Input: dimensioned drawing with shaded views. Units: mm. Origin: part minimum x, y, z. A direction names the side the tool comes from. Give positions to 0.01 mm unless a question says otherwise; leave off trailing zeros. Order: outer loops, then holes, each group sorted by start corner. A loop starts at its lowest first (then second) coordinate and runs counter-clockwise, first axis right, second up. Notation, with made-up numbers: (73, 58.5) - (117, 58.5) arc R25 cw to (117, 97.5) - close; hole circle Ø4 at (-14, 19.5). An arc over 180 degrees is marked (long way). Use a Markdown table: item, result.
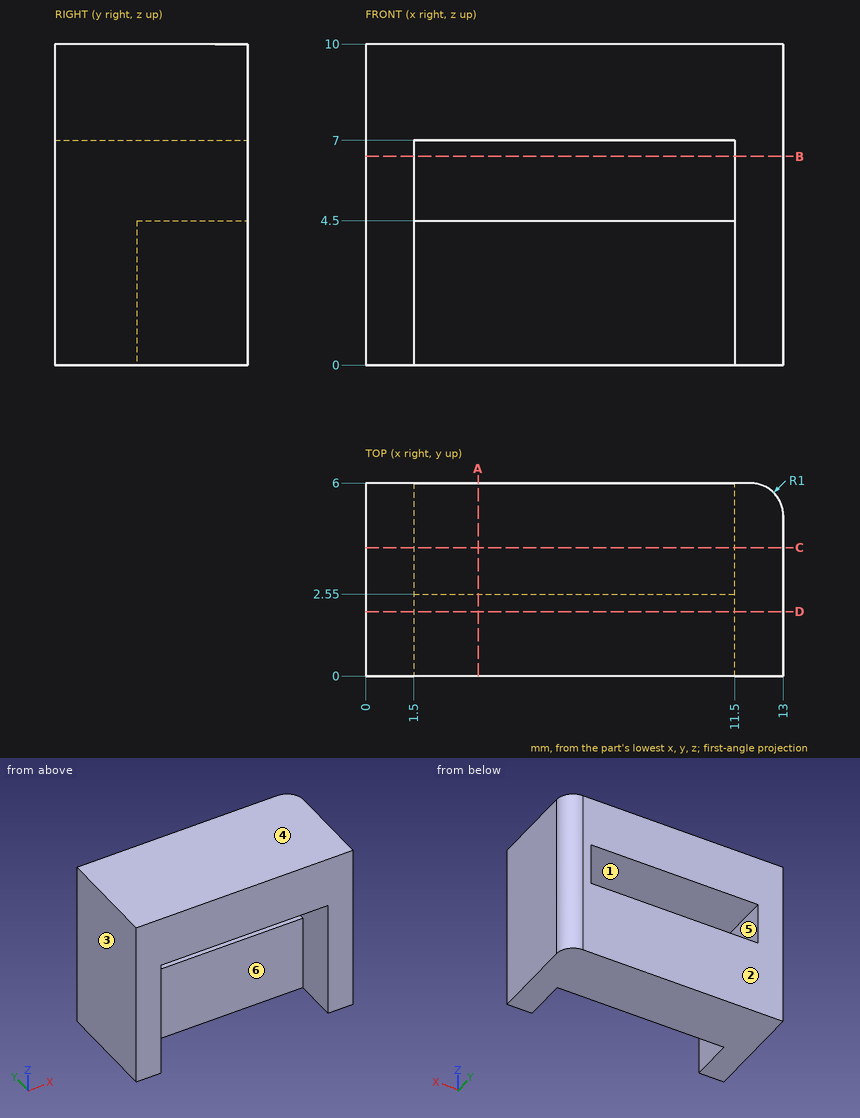
1. Section query C-C (y = 4). Return loops of the section in (x, z).
Response:
| item | result |
|---|---|
| outline | (0, 0) - (13, 0) - (13, 10) - (0, 10) - close; hole (1.5, 4.5) - (11.5, 4.5) - (11.5, 7) - (1.5, 7) - close |
2. Material intervals for line 1 along X through (y, z) = (3.5, 5.25); line 2 along Z through (x, y) = (3.75, 5.5); line 3 along Z through (x, y) = (2, 1.5), sorted ascending.
Response:
| item | result |
|---|---|
| line 1 | x = 0 to 1.5, 11.5 to 13 |
| line 2 | z = 0 to 4.5, 7 to 10 |
| line 3 | z = 7 to 10 |
3. Mould query, pull axis X, two halves, no side actions, for the marked faces 1, 2 and 3. Classes: pulls with the +X half, pulls with the -X half, needs draft (parallel to the pull), parting line crosses it, or undercut.
Response:
| item | result |
|---|---|
| face 1 | undercut |
| face 2 | needs draft |
| face 3 | pulls with the -X half |
4. Pin query (flat end, axial travel): pin 1 (2 mm diameter, centred on x = 7.5, z = 3, fed in from -Y); pin 2 (1.8 mm diameter, centred on y = 4, z = 5, fed in from -X). Return the tip coordinate at first contact, or that it passes through.
Response:
| item | result |
|---|---|
| pin 1 | stops at y = 2.55 |
| pin 2 | stops at x = 0 |
5. Section query A-A (x = 3.5). Return loops of the section in (y, z).
Response:
| item | result |
|---|---|
| outline | (0, 7) - (6, 7) - (6, 10) - (0, 10) - close; (2.55, 0) - (6, 0) - (6, 4.5) - (2.55, 4.5) - close |
6. Section query B-B (z = 6.5). Return loops of the section in (x, y), then the cut area to 3 significant figures.
Response:
| item | result |
|---|---|
| outline | (0, 0) - (1.5, 0) - (1.5, 6) - (0, 6) - close; (11.5, 0) - (13, 0) - (13, 5) arc R1 ccw to (12, 6) - (11.5, 6) - close |
| area | 17.8 mm^2 |
7. Set-up query: the marked faces 4, 5 and 6. Return all of +Z, -Z, +X, -X, +Y, -Y with unobstructed straight access to the full face (end or side cutting, diameter ignored); none if empty.
Response:
| item | result |
|---|---|
| face 4 | +Z, +X, -X, +Y, -Y |
| face 5 | -Y |
| face 6 | -Z, -Y |
8. Section query D-D (y = 2). Return loops of the section in (x, z), then the cut area to 3 significant figures.
Response:
| item | result |
|---|---|
| outline | (0, 0) - (1.5, 0) - (1.5, 7) - (11.5, 7) - (11.5, 0) - (13, 0) - (13, 10) - (0, 10) - close |
| area | 60.0 mm^2 |
